```python
from build123d import *

# Parameters (mm, degrees)
F0_W          = 63
F0_H          = 30
F1_DEPTH      = 2
F2_T1_DEPTH   = 65.5
F3_W          = 32
F3_H          = 24
F4_DEPTH      = 25
F5_R          = 10
F7_E2_W       = 32.4974397272
F7_E2_H       = 2
F7_E3_0_1_0_W = 32.4974397272
F7_E3_0_1_0_H = 2
F7_E3_0_2_0_W = 32.4974397272
F7_E3_0_2_0_H = 2
F7_E3_0_3_0_W = 32.4974397272
F7_E3_0_3_0_H = 2
F7_E3_0_4_0_W = 32.4974397272
F7_E3_0_4_0_H = 2
F7_E3_0_5_0_W = 32.4974397272
F7_E3_0_5_0_H = 2
F7_E3_0_6_0_W = 32.4974397272
F7_E3_0_6_0_H = 2
F8_DEPTH      = 0.5


# Not quite as in the source:
# - a fillet or chamfer that OpenCascade refuses, or shapes differently, is made with other operations: its cross-section is extruded or revolved along the edge and cut away or added


with BuildPart() as f1:
    # F0 (on Top) → F1 (new body)
    with BuildSketch(Plane.XY):
        Rectangle(F0_W, F0_H)
    extrude(amount=F1_DEPTH)

    # F2: fillet of radius 12.7 on 2 edges, made by hand

    # F2_s2 → F2_t1 (cut)
    with BuildSketch(Plane.XY.offset(-31.75)):
        with BuildLine():
            add(Edge.make_bspline(
                [(-18.8, 15), (-31.5, 15), (-31.5, 2.3)],
                knots=[0, 0, 0, 1, 1, 1], degree=2, weights=[1, 0.9230769231, 1]))
            Line((-31.5, 2.3), (-31.5, 15))
            Line((-31.5, 15), (-18.8, 15))
        make_face()
        with BuildLine():
            add(Edge.make_bspline(
                [(-31.5, -2.3), (-31.5, -15), (-18.8, -15)],
                knots=[0, 0, 0, 1, 1, 1], degree=2, weights=[1, 0.9230769231, 1]))
            Line((-18.8, -15), (-31.5, -15))
            Line((-31.5, -15), (-31.5, -2.3))
        make_face()
    extrude(amount=F2_T1_DEPTH, mode=Mode.SUBTRACT)

    # F3 (on face) → F4 (cut)
    with BuildSketch(Plane.XY.offset(2)):
        with Locations((-11.5, 0)):
            Rectangle(F3_W, F3_H)
    extrude(amount=-F4_DEPTH, mode=Mode.SUBTRACT)

    # F5
    f5_edges = [f1.edges().sort_by_distance(p)[0] for p in [
        (-27.5, 12, 1),
        (-27.5, -12, 1),
    ]]
    fillet(f5_edges, radius=F5_R)

    # F7_E2 (on explicit) + F7_E3_0_1_0 (on explicit) + F7_E3_0_2_0 (on explicit) + F7_E3_0_3_0 (on explicit) + F7_E3_0_4_0 (on explicit) + F7_E3_0_5_0 (on explicit) + F7_E3_0_6_0 (on explicit) → F8 (join, symmetric)
    with BuildSketch(Plane(origin=(4.5, -9, 2), x_dir=(-1, 0, 0), z_dir=(0, -1, 0))):
        with Locations((16.2487198636, 1)):
            Rectangle(F7_E2_W, F7_E2_H)
    with BuildSketch(Plane(origin=(4.5, -6, 2), x_dir=(-1, 0, 0), z_dir=(0, -1, 0))):
        with Locations((16.2487198636, 1)):
            Rectangle(F7_E3_0_1_0_W, F7_E3_0_1_0_H)
    with BuildSketch(Plane(origin=(4.5, -3, 2), x_dir=(-1, 0, 0), z_dir=(0, -1, 0))):
        with Locations((16.2487198636, 1)):
            Rectangle(F7_E3_0_2_0_W, F7_E3_0_2_0_H)
    with BuildSketch(Plane(origin=(4.5, 0, 2), x_dir=(-1, 0, 0), z_dir=(0, -1, 0))):
        with Locations((16.2487198636, 1)):
            Rectangle(F7_E3_0_3_0_W, F7_E3_0_3_0_H)
    with BuildSketch(Plane(origin=(4.5, 3, 2), x_dir=(-1, 0, 0), z_dir=(0, -1, 0))):
        with Locations((16.2487198636, 1)):
            Rectangle(F7_E3_0_4_0_W, F7_E3_0_4_0_H)
    with BuildSketch(Plane(origin=(4.5, 6, 2), x_dir=(-1, 0, 0), z_dir=(0, -1, 0))):
        with Locations((16.2487198636, 1)):
            Rectangle(F7_E3_0_5_0_W, F7_E3_0_5_0_H)
    with BuildSketch(Plane(origin=(4.5, 9, 2), x_dir=(-1, 0, 0), z_dir=(0, -1, 0))):
        with Locations((16.2487198636, 1)):
            Rectangle(F7_E3_0_6_0_W, F7_E3_0_6_0_H)
    extrude(amount=F8_DEPTH, both=True)


solid = f1.part
```
Geometry check sheet. Reference: the model listing, model coordinates, mm. Coordinates: 2 decimals unless noted, no trailing zeros. One line per item, written item: value. Start each with the question number.
(1) Cross-section at A-A on x = -7. Count the separate pieces of the cut face and the enclosed holes in it, plus the area to 3 significant figures.
(2) Material ranges on line 1 (X direction, y = 1.5, z = 1.2); line 2 (X direction, y = 3, z = 1.55); line 3 (X direction, y = -11, z = 0.4), recorded low to high. Write a range as [from, to].
(3) Mould release check, pull along Y, two halves, no side actions. Record for faces 1 (the flat face through (-31.5, 0, 1)), 2 (the flat face through (-11, 3.5, 1)), 3 (the flat face through (6, -15, 1)): released by +Y, released by -Y, zero draft, split by the parting line, or undercut.
(4) Depth check by flat-ended pin: P1, Ø0.6, axis at y = -7.5, z = 1, coming from the -X side; P2, Ø0.6, axis at y = 5, z = 1, coming from the -X side; P3, Ø0.6, axis at y = -10.5, z = 1.5, coming from the -X side. Enter the tip coordinate at first touch or a pass-through.
Results below:
1. separate pieces: 9
1. enclosed holes: 0
1. area: 26.0 mm2
2. line 1: x = [-31.5, -27.5], [4.5, 31.5]
2. line 2: x = [-31.49, 31.5]
2. line 3: x = [-28.83, -21.86], [4.5, 31.5]
3. face 1: zero draft
3. face 2: undercut
3. face 3: released by -Y
4. P1: stops at x = -30.83
4. P2: stops at x = -31.36
4. P3: stops at x = -29.43
